Check sheet for the drawn part. Datum: minimum x, y, z corner. Units: mm. A direction names the side the tool comes from. Coordinates: 2 decimals unless noted, no trailing zeros. Order: outer loops, then holes, each group sorted by start corner. A loop starts at its lowest first (then second) coordinate and runs counter-clockwise, first axis right, second up.
1. Set-up check for the marked faces 4 and 5: record each of +Z, -Z, +X, -X, +Y, -Y from which the full face is reachable in a straight line by a thin tool's end or side.
2. Cross-section at A-A (z = 28). Enter the section's corners in (x, y).
3. Cross-section at C-C (z = 19). Enter the section's corners in (x, y), then the cut area to 3 significant figures.
4. Cross-section at B-B (x = 87.5). Enter the section's corners in (y, z), then the cut area to 3 significant figures.
5. Gauge pin test, flat ends, axial feed: pin 1 Ø10 at (y, z) = (26.5, 13.5) entering from -X; pin 2 Ø1 at (y, z) = (135, 23) entering from +X; pin 3 Ø2.5 at (x, z) = (11.5, 1.5) entering from -Y. Record the tip position at first contact, or that the pin passes through.
6. Cross-section at D-D (y = 10). Enter the section's corners in (x, z).
7. Draft check along Y on the marked faces 1, 2 and 3. Enter one of: released by +Y, released by -Y, zero draft, split by the parting line, or undercut.
8. Thickness scan on line 1 (X direction, y = 140, z = 0.9); line 2 (X direction, y = 118.5, z = 36); line 3 (X direction, y = 158.25, z = 28). Record the ranges inside material, lowest first.
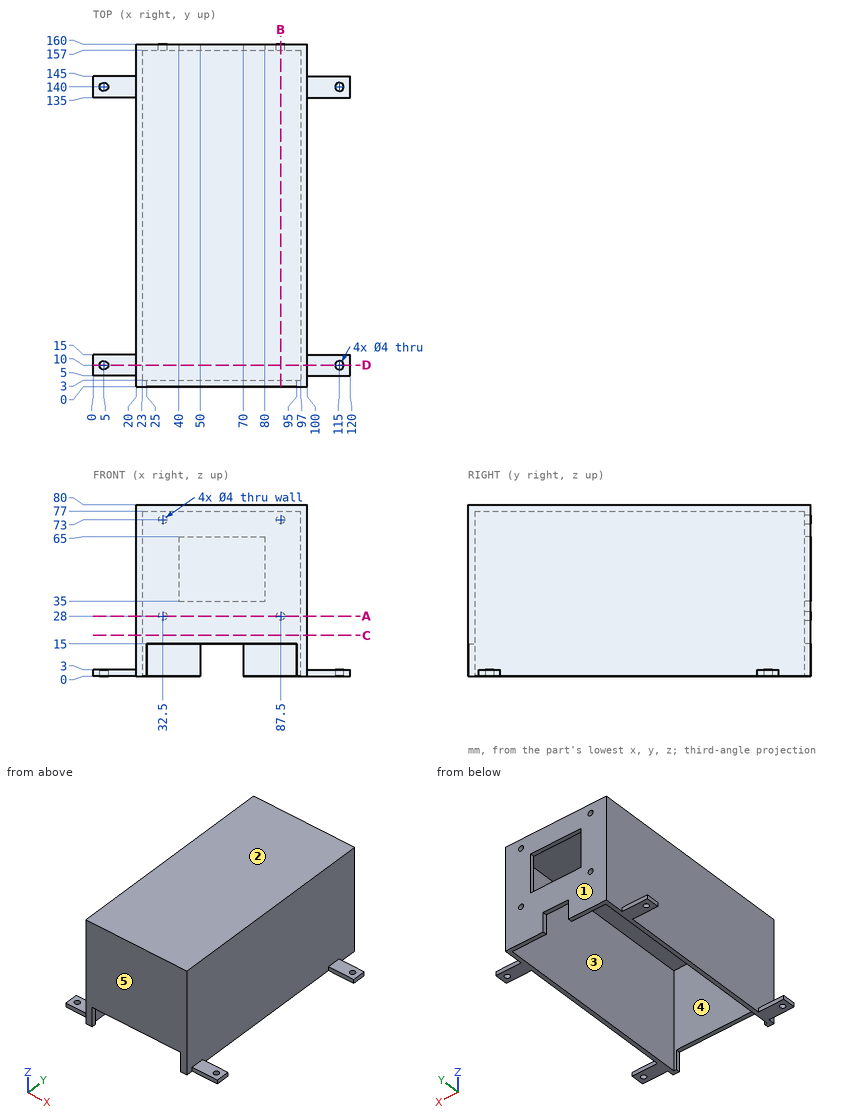
Data:
1. face 4: -Z
1. face 5: +Z, -Z, +X, -X, -Y
2. outline: (20, 0) - (100, 0) - (100, 160) - (89.5, 160) - (89.5, 157) - (97, 157) - (97, 3) - (23, 3) - (23, 157) - (30.5, 157) - (30.5, 160) - (20, 160) - close; (34.5, 157) - (85.5, 157) - (85.5, 160) - (34.5, 160) - close
3. outline: (20, 0) - (100, 0) - (100, 160) - (20, 160) - close; hole (23, 3) - (97, 3) - (97, 157) - (23, 157) - close
3. area: 1,400 mm2
4. outline: (0, 15) - (3, 15) - (3, 77) - (157, 77) - (157, 75) - (160, 75) - (160, 80) - (0, 80) - close; (157, 0) - (160, 0) - (160, 26) - (157, 26) - close; (157, 30) - (160, 30) - (160, 71) - (157, 71) - close
4. area: 873 mm2
5. pin 1: stops at x = 20
5. pin 2: stops at x = 100
5. pin 3: stops at y = 5
6. outline: (0, 0) - (3, 0) - (3, 3) - (0, 3) - close; (7, 0) - (23, 0) - (23, 77) - (97, 77) - (97, 0) - (113, 0) - (113, 3) - (100, 3) - (100, 80) - (20, 80) - (20, 3) - (7, 3) - close; (117, 0) - (120, 0) - (120, 3) - (117, 3) - close
7. face 1: released by +Y
7. face 2: zero draft
7. face 3: undercut
8. line 1: x = 0 to 3, 7 to 23, 97 to 113, 117 to 120
8. line 2: x = 20 to 23, 97 to 100
8. line 3: x = 20 to 30.5, 34.5 to 85.5, 89.5 to 100
